Geometry: final body of the model. Coordinates: model frame, mm. Coordinates: 2 decimals unless noted, no trailing zeros. Order: outer loops, then holes, each group sorted by start corner. A loop starts at its lowest first (then second) coordinate and runs counter-clockwise, first axis right, second up. Notation, with made-up numbers: M 18,43.25 L 47,43.25 A25 cw 47,58.25 Z; hole C 21,-5 d4. An arc over 180 degrees is marked long. Write item = value, one per line.
from build123d import *

# Parameters (mm, degrees)
F1_DEPTH = 300
F2_SIZE  = 20


with BuildPart() as f1:
    # F0 (on Front) → F1 (new body)
    with BuildSketch(Plane.XZ):
        Polygon((0, -343.945524), (0, 0), (-125, 0), (-329.209394, -343.945524), align=None)
        Polygon((125, 0), (0, 0), (0, -343.945524), (329.209394, -343.945524), align=None)
    extrude(amount=F1_DEPTH)

    # F2
    f2_edges = [f1.edges().sort_by_distance(p)[0] for p in [
        (0, 0, -343.945524),
        (227.104697, 0, -171.972762),
        (0, 0, 0),
        (-227.104697, 0, -171.972762),
    ]]
    chamfer(f2_edges, length=F2_SIZE)


solid = f1.part
1) Section B-B, the plane z = -302. Return loops of the section in (x, y).
Numbers:
outline = M -304.31,-300 L 304.31,-300 L 304.31,-20 L 281.05,0 L -281.05,0 L -304.31,-20 Z
2) Section C-C, the plane y = -158. Return loops of the section in (x, z), and give its area (3 significant figures).
Numbers:
outline = M -329.21,-343.95 L 329.21,-343.95 L 125,0 L -125,0 Z
area = 156,000 mm²
3) Line query: L1, parallel to Z at x = -160, y = -149; L2, parallel to Z at x = -172, y = -18; L3, parallel to X at y = -170.5, z = -304. Output: solid intervals per line, ascending.
Numbers:
L1 = -343.95 to -58.95
L2 = -341.95 to -83.08
L3 = -305.49 to 305.49
4) Section A-A, the plane x = 134. Return loops of the section in (y, z), and give its area (3 significant figures).
Numbers:
outline = M -300,-343.95 L -20,-343.95 L 0,-323.95 L 0,-54.33 L -20,-15.16 L -300,-15.16 Z
area = 98,000 mm²
5) Pin query (flat end, axial travel): pin 1 (4 mm diameter, centred on x = -230, y = -232, fed in from +Z); pin 2 (4 mm diameter, centred on y = -124.5, z = -149, fed in from -X). Return the tip coordinate at first contact, or that it passes through.
Numbers:
pin_1 = -173.48
pin_2 = -214.65
